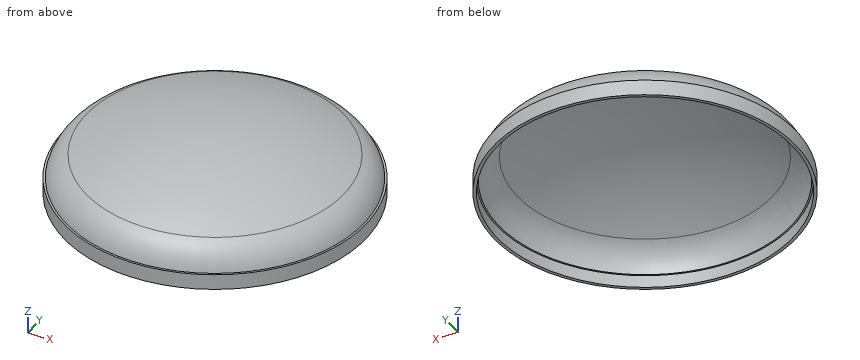
```python
from build123d import *


with BuildPart() as f1:
    # F0 (on Right) → F1 (revolve)
    with BuildSketch(Plane.YZ):
        with BuildLine():
            ThreePointArc((0, 9), (20.988092, 6.72353), (41, 0))
            ThreePointArc((41, 0), (45.010989, -3.241758), (47, -8))
            Line((47, -8), (47.5, -8))
            Line((47.5, -8), (47.5, -12))
            Line((47.5, -12), (48.5, -12))
            Line((48.5, -12), (48.5, -7))
            Line((48.5, -7), (47.828647, -7))
            ThreePointArc((47.828647, -7), (45.544324, -2.299803), (41.418842, 0.908059))
            ThreePointArc((41.418842, 0.908059), (21.202499, 7.700274), (0, 10))
            Line((0, 10), (0, 9))
        make_face()
    revolve(axis=Axis((0, 0, 4.5), (0, 0, 1)))


solid = f1.part
```
Check sheet for the modelled part. Datum: model origin and axes. Units: mm. Coordinates: 2 decimals unless noted, no trailing zeros. Order: outer loops, then holes, each group sorted by start corner. A loop starts at its lowest first (then second) coordinate and runs counter-clockwise, first axis right, second up. Notation, with made-up numbers: (-31, -30) -> (14, -30) arc R21 cw to (14, -17) -> close; hole circle Ø4 at (31.5, -0.75). An arc over 180 degrees is marked (long way). Write each question's results on one line, items separated by ' | '. Start each with the question number.
1) Material ranges on line 1 along X through (y, z) = (0, -9.5); line 2 along Y through (x, z) = (42, -9.75), recorded low to high.
2) Depth check by flat-ended pin: pin 1 (12 mm diameter, centred on x = 37.5, y = -35.5, fed in from -Z); pin 2 (10 mm diameter, centred on x = 14, z = -8.5, fed in from -Y); pin 3 (5 mm diameter, centred on x = 17.5, y = 31.5, fed in from -Z); pin 4 (2 mm diameter, centred on x = -23.5, y = 25.5, fed in from +Z). Enter the tip coordinate at first touch or a pass-through.
3) Section check A-A (z = -10). Enter the section's corners in (x, y).
Checked values:
1) line 1: -48.5 to -47.5, 47.5 to 48.5 | line 2: -24.25 to -22.19, 22.19 to 24.25
2) pin 1: z = -12 | pin 2: y = -47.66 | pin 3: z = 1.1 | pin 4: z = 4.09
3) outline: circle Ø97 at (0, 0); hole circle Ø95 at (0, 0)
